Design review of the part built by this model. Coordinates are the model's own, in mm. Face numbers are marked on the shaded views. Coordinates: 2 decimals unless noted, no trailing zeros. Write each loop counter-clockwise with the first axis right and the second up, starting at its lowest first coordinate (ties: lowest second). Pieces come first, ordered by that corner, then holes.
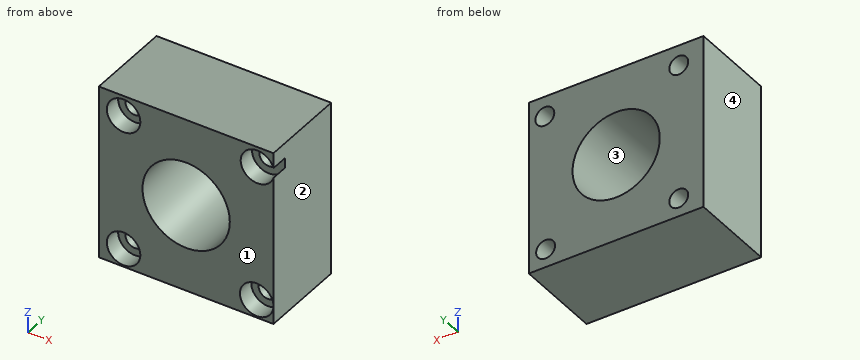
```python
from build123d import *

# Parameters (mm, degrees)
F0_W           = 50.8
F0_H           = 50.8
F1_DEPTH       = 25.4
F2_R           = 12.7
F3_DEPTH       = 25.401
F5_D           = 5.5
F5_CBORE_D     = 9.75
F5_CBORE_DEPTH = 5


with BuildPart() as f1:
    # F0 (on Front) → F1 (new body)
    with BuildSketch(Plane.XZ):
        with Locations((25.4, 25.4)):
            Rectangle(F0_W, F0_H)
    extrude(amount=F1_DEPTH)

    # F2 (on face) → F3 (cut, through all)
    with BuildSketch(Plane.XZ.offset(25.4)):
        with Locations((25.4, 25.4)):
            Circle(F2_R)
    extrude(amount=-F3_DEPTH, mode=Mode.SUBTRACT)

    # F5 (through all)
    with Locations(Plane.XZ.offset(25.4)):
        with Locations((7.1971733123, 44.9103601277), (46.1442172527, 44.9103601277), (45.92083022, 5.3215231746), (7.1971733123, 5.3215231746)):
            CounterBoreHole(F5_D / 2, F5_CBORE_D / 2, F5_CBORE_DEPTH)


solid = f1.part
```
(1) Consider section B-B (z = 25.4). Give the boundary of the cut face in (x, y), plus the area to 3 significant figures.
(2) Consider section A-A (x = 25.4). Give the boundary of the cut face in (y, z), plus the area to 3 significant figures.
(3) Insertion check: pin 1 Ø6 at (x, z) = (7.2, 44.91) entering from -Y. The pin has a flat end and moves straight along its axis. Give the tip position at first contact, or say it passes through.
(4) Wall thickness on line 1 (Z direction, x = 25.4, y = -13); line 2 (Z direction, x = 46.5, y = -16.25); line 3 (X direction, y = -2, z = 5): over which ranges is each line inside the solid? List them lowest first.
(5) Mouldability with a two-part tool opening along X and no side actions: class the marked faces 1, 2, 3 and 4 as +X half, -X half, draft (parallel to the pull), parting line (faces both ways), or undercut.
(6) Consider section C-C (y = -14). Give the boundary of the cut face in (x, z).
Results:
1. outline: (0, -25.4) - (12.7, -25.4) - (12.7, 0) - (0, 0) - close; (38.1, -25.4) - (50.8, -25.4) - (50.8, 0) - (38.1, 0) - close
1. area: 645 mm2
2. outline: (-25.4, 0) - (0, 0) - (0, 12.7) - (-25.4, 12.7) - close; (-25.4, 38.1) - (0, 38.1) - (0, 50.8) - (-25.4, 50.8) - close
2. area: 645 mm2
3. pin 1: stops at y = -20.4
4. line 1: z = 0 to 12.7, 38.1 to 50.8
4. line 2: z = 0 to 2.63, 8.01 to 42.18, 47.64 to 50.8
4. line 3: x = 0 to 4.47, 9.93 to 43.19, 48.65 to 50.8
5. face 1: draft
5. face 2: +X half
5. face 3: undercut
5. face 4: -X half
6. outline: (0, 0) - (50.8, 0) - (50.8, 50.8) - (0, 50.8) - close; hole circle Ø5.5 at (7.2, 5.32); hole circle Ø5.5 at (7.2, 44.91); hole circle Ø25.4 at (25.4, 25.4); hole circle Ø5.5 at (45.92, 5.32); hole circle Ø5.5 at (46.14, 44.91)
